For this review, take the finished solid that the model builds, in its own axes (mm). Coordinates: 2 decimals unless noted, no trailing zeros. Write each loop counter-clockwise with the first axis right and the second up, starting at its lowest first coordinate (ties: lowest second). Pieces come first, ordered by that corner, then holes.
1) To check wall thickness, follow line 1 along X through (y, z) = (0.7, -57.5) (1 decimal); line 2 along Z through (x, y) = (16, 0.7); line 3 along Z through (x, y) = (35.5, 1.35). State the ranges of each line that lie inside material, in increasing order.
2) We need section B-B on x = 22.5. Write out the cut boundary in (y, z), then the cut area to 3 significant figures.
3) Insertion check: P1, Ø1, axis at y = 0.5, z = -23.5, coming from the -X side. The pin has a flat end and moves straight along its axis. Give the tip position at first contact, or say it passes through.
4) We need section D-D on y = 0.35. Give the number of separate pieces and of enclosed holes in the cut face, then the cut area to 3 significant figures.
5) Mouldability with a two-part tool opening along Z and no side actions: class faces 1 (the face through (50, 2, -54)), 2 (the face through (5.665, 1.014, -3.594)), 3 (the face through (77.062, 1.014, -102.977)) as pulls with the +Z half, pulls with the -Z half, needs draft (parallel to the pull), parting line crosses it, or undercut.
6) We need section A-A on z = -4.4. Write out the cut boundary in (x, y) (3 decimals), then the cut area to 3 significant figures.
7) We need section C-C on x = 4.4. Write out the cut boundary in (y, z).
from build123d import *

# Parameters (mm, degrees)
SKETCH1_W           = 82.375
SKETCH1_H           = 106.187
ACRYLIC_SHEET_DEPTH = 2
SKETCH2_R           = 1.5
SKETCH2_W           = 14.1
SKETCH2_H           = 14.1
SKETCH2_W_2         = 29.7
SKETCH2_H_2         = 12.2
ACRYLIC_CUT_DEPTH   = 135.407289959


with BuildPart() as part:
    # Sketch1 → Acrylic-Sheet (new body)
    with BuildSketch(Plane(origin=(0, 0, 0), x_dir=(1, 0, 0), z_dir=(0, 1, 0))):
        with Locations((41.1875, 53.0935)):
            Rectangle(SKETCH1_W, SKETCH1_H)
    extrude(amount=ACRYLIC_SHEET_DEPTH)

    # Sketch2 → Acrylic-Cut (cut, through all)
    with BuildSketch(Plane(origin=(0, 2, 0), x_dir=(1, 0, 0), z_dir=(0, 1, 0))):
        with Locations(Location((4.4, 101.787, 0), (0, 0, 270))):
            Circle(SKETCH2_R)
        with Locations(Location((77.975, 101.787, 0), (0, 0, 270))):
            Circle(SKETCH2_R)
        with Locations(Location((77.975, 4.4, 0), (0, 0, 270))):
            Circle(SKETCH2_R)
        with Locations(Location((4.4, 4.4, 0), (0, 0, 270))):
            Circle(SKETCH2_R)
        with Locations((22.1375, 60.2375)):
            Rectangle(SKETCH2_W, SKETCH2_H)
        with Locations((27.45, 80.587)):
            Rectangle(SKETCH2_W_2, SKETCH2_H_2)
        with Locations((41.1875, 60.2375)):
            Rectangle(SKETCH2_W, SKETCH2_H)
        with Locations((60.2375, 60.2375)):
            Rectangle(SKETCH2_W, SKETCH2_H)
        with Locations((22.1375, 41.1875)):
            Rectangle(SKETCH2_W, SKETCH2_H)
        with Locations((41.1875, 41.1875)):
            Rectangle(SKETCH2_W, SKETCH2_H)
        with Locations((60.2375, 41.1875)):
            Rectangle(SKETCH2_W, SKETCH2_H)
        with Locations((31.6625, 22.1375)):
            Rectangle(SKETCH2_W, SKETCH2_H)
        with Locations((60.2375, 22.1375)):
            Rectangle(SKETCH2_W, SKETCH2_H)
    extrude(amount=-ACRYLIC_CUT_DEPTH, mode=Mode.SUBTRACT)


solid = part.part
Result:
1. line 1: x = 0 to 15.1, 29.2 to 34.1, 48.2 to 53.2, 67.3 to 82.4
1. line 2: z = -106.19 to -86.69, -74.49 to -67.29, -53.19 to -48.24, -34.14 to 0
1. line 3: z = -106.19 to -86.69, -74.49 to -67.29, -53.19 to -48.24, -34.14 to -29.19, -15.09 to 0
2. outline: (0, -106.19) - (2, -106.19) - (2, -86.69) - (0, -86.69) - close; (0, -74.49) - (2, -74.49) - (2, -67.29) - (0, -67.29) - close; (0, -53.19) - (2, -53.19) - (2, -48.24) - (0, -48.24) - close; (0, -34.14) - (2, -34.14) - (2, 0) - (0, 0) - close
2. area: 132 mm2
3. P1: stops at x = 0
4. separate pieces: 1
4. enclosed holes: 13
4. area: 6,770 mm2
5. face 1: needs draft
5. face 2: undercut
5. face 3: undercut
6. outline: (0, 0) - (2.9, 0) - (2.9, 2) - (0, 2) - close; (5.9, 0) - (76.475, 0) - (76.475, 2) - (5.9, 2) - close; (79.475, 0) - (82.375, 0) - (82.375, 2) - (79.475, 2) - close
6. area: 153 mm2
7. outline: (0, -106.19) - (2, -106.19) - (2, -103.29) - (0, -103.29) - close; (0, -100.29) - (2, -100.29) - (2, -5.9) - (0, -5.9) - close; (0, -2.9) - (2, -2.9) - (2, 0) - (0, 0) - close
